Geometry: final body of the model. Coordinates: model frame, mm. A direction names the side the tool comes from. Give positions to 0.01 mm unless a question says otherwise; leave off trailing zeros. Loops run counter-clockwise (first coordinate to the right, second up) from the corner with the lowest first, then second, coordinate; pieces in that order, holes last.
from build123d import *

# Parameters (mm, degrees)
IZIM1_R                     = 350
Y_KSEKLIK_EKSTR_ZYON1_DEPTH = 5


with BuildPart() as part:
    # Çizim1 → Yükseklik-Ekstrüzyon1 (new body)
    # profile 1 of 7: a face of its own
    with BuildSketch(Plane(origin=(0, 0, 0), x_dir=(1, 0, 0), z_dir=(0, 1, 0))):
        with Locations(Location((0, 0, 0), (0, 0, 270))):
            Circle(IZIM1_R)
        with BuildLine():
            ThreePointArc((70.062926922, 71.352549156), (75.892103529, 65.118266423), (81.168439698, 58.409625893))
            Line((81.168439698, 58.409625893), (168.205080757, 108.660254038))
            Line((168.205080757, 108.660254038), (178.205080757, 91.339745962))
            Line((178.205080757, 91.339745962), (91.168439698, 41.089117818))
            ThreePointArc((91.168439698, 41.089117818), (94.340124737, 33.165356392), (96.824583655, 25))
            Line((96.824583655, 25), (150, 55.700840941))
            Line((150, 55.700840941), (150, -55.700840941))
            Line((150, -55.700840941), (96.824583655, -25))
            ThreePointArc((96.824583655, -25), (94.340124737, -33.165356392), (91.168439698, -41.089117817))
            Line((91.168439698, -41.089117817), (178.205080757, -91.339745962))
            Line((178.205080757, -91.339745962), (168.205080757, -108.660254038))
            Line((168.205080757, -108.660254038), (81.168439698, -58.409625893))
            ThreePointArc((81.168439698, -58.409625893), (75.892103529, -65.118266423), (70.062926922, -71.352549156))
            Line((70.062926922, -71.352549156), (123.238343267, -102.053390097))
            Line((123.238343267, -102.053390097), (26.761656733, -157.754231038))
            Line((26.761656733, -157.754231038), (26.761656733, -96.352549156))
            ThreePointArc((26.761656733, -96.352549156), (18.448021208, -98.283622814), (10, -99.498743711))
            Line((10, -99.498743711), (10, -200))
            Line((10, -200), (-10, -200))
            Line((-10, -200), (-10, -99.498743711))
            ThreePointArc((-10, -99.498743711), (-18.448021208, -98.283622814), (-26.761656733, -96.352549156))
            Line((-26.761656733, -96.352549156), (-26.761656733, -157.754231038))
            Line((-26.761656733, -157.754231038), (-123.238343267, -102.053390097))
            Line((-123.238343267, -102.053390097), (-70.062926922, -71.352549156))
            ThreePointArc((-70.062926922, -71.352549156), (-75.892103529, -65.118266423), (-81.168439698, -58.409625893))
            Line((-81.168439698, -58.409625893), (-168.205080757, -108.660254038))
            Line((-168.205080757, -108.660254038), (-178.205080757, -91.339745962))
            Line((-178.205080757, -91.339745962), (-91.168439698, -41.089117817))
            ThreePointArc((-91.168439698, -41.089117817), (-94.340124737, -33.165356392), (-96.824583655, -25))
            Line((-96.824583655, -25), (-150, -55.700840941))
            Line((-150, -55.700840941), (-150, 55.700840941))
            Line((-150, 55.700840941), (-96.824583655, 25))
            ThreePointArc((-96.824583655, 25), (-94.340124737, 33.165356392), (-91.168439698, 41.089117818))
            Line((-91.168439698, 41.089117818), (-178.205080757, 91.339745962))
            Line((-178.205080757, 91.339745962), (-168.205080757, 108.660254038))
            Line((-168.205080757, 108.660254038), (-81.168439698, 58.409625893))
            ThreePointArc((-81.168439698, 58.409625893), (-75.892103529, 65.118266423), (-70.062926922, 71.352549156))
            Line((-70.062926922, 71.352549156), (-123.238343267, 102.053390097))
            Line((-123.238343267, 102.053390097), (-26.761656733, 157.754231038))
            Line((-26.761656733, 157.754231038), (-26.761656733, 96.352549156))
            ThreePointArc((-26.761656733, 96.352549156), (-18.448021208, 98.283622814), (-10, 99.498743711))
            Line((-10, 99.498743711), (-10, 200))
            Line((-10, 200), (10, 200))
            Line((10, 200), (10, 99.498743711))
            ThreePointArc((10, 99.498743711), (18.448021208, 98.283622814), (26.761656733, 96.352549156))
            Line((26.761656733, 96.352549156), (26.761656733, 157.754231038))
            Line((26.761656733, 157.754231038), (123.238343267, 102.053390097))
            Line((123.238343267, 102.053390097), (70.062926922, 71.352549156))
        make_face(mode=Mode.SUBTRACT)
    # profile 2 of 7: a face of its own
    with BuildSketch(Plane(origin=(0, 0, 0), x_dir=(1, 0, 0), z_dir=(0, 1, 0))):
        with BuildLine():
            Line((-26.761656733, -157.754231038), (-26.761656733, -96.352549156))
            ThreePointArc((-26.761656733, -96.352549156), (-50, -86.602540378), (-70.062926922, -71.352549156))
            Line((-70.062926922, -71.352549156), (-123.238343267, -102.053390097))
            Line((-123.238343267, -102.053390097), (-26.761656733, -157.754231038))
        make_face()
    # profile 3 of 7: a face of its own
    with BuildSketch(Plane(origin=(0, 0, 0), x_dir=(1, 0, 0), z_dir=(0, 1, 0))):
        with BuildLine():
            ThreePointArc((-96.824583655, -25), (-100, 0), (-96.824583655, 25))
            Line((-96.824583655, 25), (-150, 55.700840941))
            Line((-150, 55.700840941), (-150, -55.700840941))
            Line((-150, -55.700840941), (-96.824583655, -25))
        make_face()
    # profile 4 of 7: a face of its own
    with BuildSketch(Plane(origin=(0, 0, 0), x_dir=(1, 0, 0), z_dir=(0, 1, 0))):
        with BuildLine():
            ThreePointArc((-70.062926922, 71.352549156), (-50, 86.602540378), (-26.761656733, 96.352549156))
            Line((-26.761656733, 96.352549156), (-26.761656733, 157.754231038))
            Line((-26.761656733, 157.754231038), (-123.238343267, 102.053390097))
            Line((-123.238343267, 102.053390097), (-70.062926922, 71.352549156))
        make_face()
    # profile 5 of 7: a face of its own
    with BuildSketch(Plane(origin=(0, 0, 0), x_dir=(1, 0, 0), z_dir=(0, 1, 0))):
        with BuildLine():
            ThreePointArc((26.761656733, 96.352549156), (50, 86.602540378), (70.062926922, 71.352549156))
            Line((70.062926922, 71.352549156), (123.238343267, 102.053390097))
            Line((123.238343267, 102.053390097), (26.761656733, 157.754231038))
            Line((26.761656733, 157.754231038), (26.761656733, 96.352549156))
        make_face()
    # profile 6 of 7: a face of its own
    with BuildSketch(Plane(origin=(0, 0, 0), x_dir=(1, 0, 0), z_dir=(0, 1, 0))):
        with BuildLine():
            Line((150, 55.700840941), (96.824583655, 25))
            ThreePointArc((96.824583655, 25), (100, 0), (96.824583655, -25))
            Line((96.824583655, -25), (150, -55.700840941))
            Line((150, -55.700840941), (150, 55.700840941))
        make_face()
    # profile 7 of 7: a face of its own
    with BuildSketch(Plane(origin=(0, 0, 0), x_dir=(1, 0, 0), z_dir=(0, 1, 0))):
        with BuildLine():
            Line((123.238343267, -102.053390097), (70.062926922, -71.352549156))
            ThreePointArc((70.062926922, -71.352549156), (50, -86.602540378), (26.761656733, -96.352549156))
            Line((26.761656733, -96.352549156), (26.761656733, -157.754231038))
            Line((26.761656733, -157.754231038), (123.238343267, -102.053390097))
        make_face()
    extrude(amount=Y_KSEKLIK_EKSTR_ZYON1_DEPTH)


solid = part.part
Item 1: Set-up query: faces 1 (the face through (125.3, 2.46, 83.89)), 2 (the face through (73, 5, 73)). Return all of +Z, -Z, +X, -X, +Y, -Y with unobstructed straight access to the full face (end or side cutting, diameter ignored); none if empty.
Values follow:
face 1: +Y, -Y
face 2: +Z, -Z, +X, -X, +Y
Item 2: Ray query, probe 1 along X at (y, z) = (0.55, -2); probe 2 along X at (y, z) = (0.2, -70.5); probe 3 along Z at (x, y) = (40, 0.8). Return the intervals inside material, ascending.
Values follow:
probe 1: x = -349.99 to -99.98, 99.98 to 349.99
probe 2: x = -342.83 to -142.11, -102.11 to -70.92, 70.92 to 102.11, 142.11 to 342.83
probe 3: z = -347.71 to -91.65, 91.65 to 347.71
Item 3: Section query B-B on x = 0. Return loops of the section in (y, z).
Values follow:
outline: (0, -350) - (5, -350) - (5, -200) - (0, -200) - close; (0, 200) - (5, 200) - (5, 350) - (0, 350) - close
Item 4: Section query A-A on z = 0. Return loops of the section in (x, y), plus the area to 3 significant figures.
Values follow:
outline: (-350, 0) - (-100, 0) - (-100, 5) - (-350, 5) - close; (100, 0) - (350, 0) - (350, 5) - (100, 5) - close
area: 2,500 mm2
Item 5: Section query C-C on x = -257. Return loops of the section in (y, z).
Values follow:
outline: (0, -237.59) - (5, -237.59) - (5, 237.59) - (0, 237.59) - close
Item 6: Pin query (flat end, axial travel): pin 1 (1 mm diameter, centred on y = 1.5, z = -143.5, fed in from +X); pin 2 (3 mm diameter, centred on x = -135.5, y = 2, fed in from +Z); pin 3 (1.5 mm diameter, centred on y = 2.5, z = 136.5, fed in from -X). Return the tip coordinate at first contact, or that it passes through.
Values follow:
pin 1: stops at x = 319.45
pin 2: stops at z = 323.33
pin 3: stops at x = -322.6
Item 7: Draft query along X for faces 3 (the face through (347.022, 2.465, -45.563)), 4 (the face through (-135.3, 2.46, 66.57)), 5 (the face through (73, 0, 73)). Return one class per face: +X half, -X half, draft (parallel to the pull), parting line (faces both ways), or undercut.
Values follow:
face 3: parting line
face 4: undercut
face 5: draft
